Here's how the part is built. I have some questions about the finished solid (model axes, mm). Face numbers are marked on the shaded views. Coordinates: 2 decimals unless noted, no trailing zeros. Write each loop counter-clockwise with the first axis right and the second up, starting at its lowest first coordinate (ties: lowest second). Pieces come first, ordered by that corner, then holes. Notation, with made-up numbers: (28.25, -9) - (69.25, -9) arc R13 ccw to (69.25, 2) - close; hole circle Ø8 at (89, -27). An arc over 180 degrees is marked (long way). Answer in a Markdown table with one row per item. Add a question column.
Item 1: Imagine slicing it at D-D (z = 15.5). Please give me the cut outline in (x, y).
Item 2: Imagine slicing it at C-C (x = 23). Please give me the cut outline in (y, z), plus the area to 3 significant figures.
Item 3: Imagine slicing it at A-A (x = 102.5). Please give me the cut outline in (y, z).
Item 4: We'd pull the mould along Z, two halves only. Please class the marked faces 1, 2 and 3: +Z half, -Z half, draft (parallel to the pull), parting line (faces both ways), or undercut.
Item 5: If I drill on probe 1 along Z at (x, y) = (6, 20); probe 2 along Y at (x, z) = (3.5, 0); probe 3 along Y at (x, z) = (4, 0), over which ranges is the centre line in solid material (lowest first)? Write a range as from..to.
Item 6: I'm going to push flat-ended pins straight in: pin 1 (4.5 mm diameter, centred on y = 20, z = 0, fed in from -X); pin 2 (8 mm diameter, centred on x = 36.5, z = 35.5, fed in from +Y); pin 3 (6 mm diameter, centred on y = 55, z = 0, fed in from +X). Where does each tip first touch, or does it pass through?
Item 7: Imagine slicing it at B-B (y = 50.5). Please give me the cut outline in (x, z), plus the area to 3 significant figures.
from build123d import *

# Parameters (mm, degrees)
BOSS_EXTRUDE1_DEPTH        = 62.5
BOSS_EXTRUDE2_DEPTH        = 5
SKETCH3_R                  = 64
CUT_EXTRUDE1_DEPTH         = 111
F_10_CLEARANCE_HOLE1_D     = 4.7752
F_10_CLEARANCE_HOLE1_DEPTH = 12.7
F_10_CLEARANCE_HOLE1_TIP   = 1.434614814


with BuildPart() as part:
    # Sketch2 → Boss-Extrude1 (new body, symmetric)
    with BuildSketch(Plane.XY):
        Polygon((0, 0), (0, 100), (125, 55), (125, 0), align=None)
    extrude(amount=BOSS_EXTRUDE1_DEPTH, both=True)

    # Sketch4 → Boss-Extrude2 (add)
    with BuildSketch(Plane.XY.offset(62.5)):
        Polygon((0, 0), (0, 110), (125, 65), (125, 0), align=None)
    boss_extrude2 = extrude(amount=BOSS_EXTRUDE2_DEPTH)

    # Mirror1: Boss-Extrude2 across plane
    add(boss_extrude2.mirror(Plane.XY))

    # Sketch3 → Cut-Extrude1 (cut, through all)
    with BuildSketch(Plane.XZ):
        with Locations((125, 0)):
            Circle(SKETCH3_R)
    extrude(amount=-CUT_EXTRUDE1_DEPTH, mode=Mode.SUBTRACT)

    # #10 Clearance Hole1
    with Locations(Plane.ZY):
        with Locations((0, 55), (0, 20)):
            Hole(F_10_CLEARANCE_HOLE1_D / 2, depth=F_10_CLEARANCE_HOLE1_DEPTH)
            with Locations((0, 0, -(F_10_CLEARANCE_HOLE1_DEPTH + F_10_CLEARANCE_HOLE1_TIP / 2))):  # 118° drill point
                Cone(0, F_10_CLEARANCE_HOLE1_D / 2, F_10_CLEARANCE_HOLE1_TIP, mode=Mode.SUBTRACT)


solid = part.part
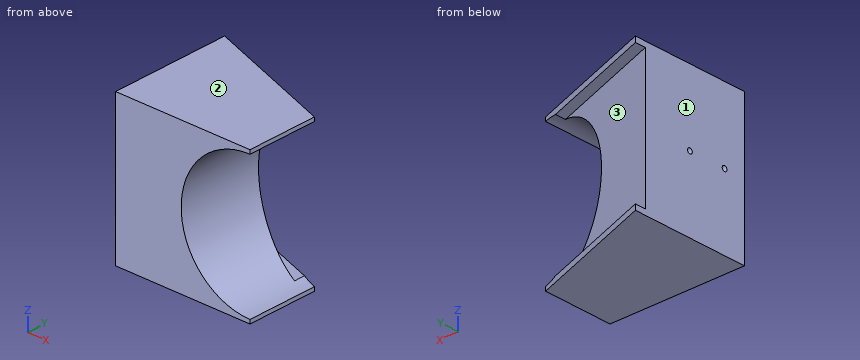
Here are the results:
| question | item | result |
|---|---|---|
| 1 | outline | (0, 0) - (62.91, 0) - (62.91, 77.35) - (0, 100) - close |
| 2 | outline | (0, -67.5) - (101.72, -67.5) - (101.72, -62.5) - (91.72, -62.5) - (91.72, 62.5) - (101.72, 62.5) - (101.72, 67.5) - (0, 67.5) - close |
| 2 | area | 12,500 mm2 |
| 3 | outline | (0, -67.5) - (73.1, -67.5) - (73.1, -62.5) - (63.1, -62.5) - (63.1, -59.91) - (0, -59.91) - close; (0, 59.91) - (63.1, 59.91) - (63.1, 62.5) - (73.1, 62.5) - (73.1, 67.5) - (0, 67.5) - close |
| 4 | face 1 | draft |
| 4 | face 2 | +Z half |
| 4 | face 3 | undercut |
| 5 | probe 1 | z = -67.5..-2.39, 2.39..67.5 |
| 5 | probe 2 | y = 0..17.61, 22.39..52.61, 57.39..98.74 |
| 5 | probe 3 | y = 0..17.61, 22.39..52.61, 57.39..98.56 |
| 6 | pin 1 | stops at x = 12.78 |
| 6 | pin 2 | stops at y = 88.3 |
| 6 | pin 3 | stops at x = 61.07 |
| 7 | outline | (0, -67.5) - (125, -67.5) - (125, -64) arc R64 cw to (125, 64) - (125, 67.5) - (0, 67.5) - close |
| 7 | area | 10,400 mm2 |
